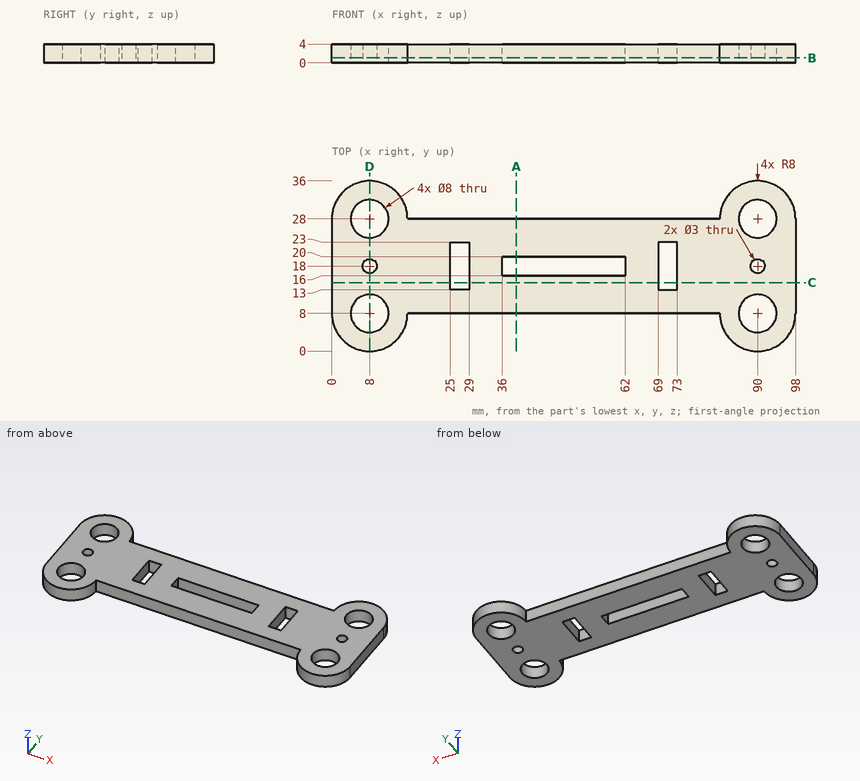
Here's the drawing with two shaded views (mm, measured from the low corner). I have some questions. Round coordinates to 2 decimals unless told otherwise and drop trailing zeros. Order: outer loops, then holes, each group sorted by start corner. A loop starts at its lowest first (then second) coordinate and runs counter-clockwise, first axis right, second up. Notation, with made-up numbers: (14, -39.5) -> (62, -39.5) arc R29 cw to (62, -5.5) -> close; hole circle Ø2 at (74.25, 51). An arc over 180 degrees is marked (long way). Return JSON: item names as keys, results as strings.
Q1. I need wall thicknesses on line 1 along X through (y, z) = (18, 2.3); line 2 along X through (y, z) = (14, 1.1); line 3 along Y through (x, z) = (8, 2.05). Which ranges of each line are inside material? Lowest first, please. Write a range as from..to.
Filled sheet:
{"line 1": "x = 0..6.5, 9.5..25, 29..36, 62..69, 73..88.5, 91.5..98", "line 2": "x = 0..25, 29..69, 73..98", "line 3": "y = 0..4, 12..16.5, 19.5..24, 32..36"}
Q2. If we section it at C-C on y = 14.5: List the corners of the cut face in (x, z) for me.
Filled sheet:
{"outline": "(0, 0) -> (25, 0) -> (25, 4) -> (0, 4) -> close; (29, 0) -> (69, 0) -> (69, 4) -> (29, 4) -> close; (73, 0) -> (98, 0) -> (98, 4) -> (73, 4) -> close"}
Q3. For pin 1 Ø1.2 at (x, z) = (26, 2.5) entering from +Y; pin 2 Ø2 at (x, z) = (71, 3) entering from -Y, each with a flat end and sliding along its axis, tell me the tip position at first contact or that it passes through.
Filled sheet:
{"pin 1": "stops at y = 28", "pin 2": "stops at y = 8"}
Q4. If we section it at D-D on x = 8: List the corners of the cut face in (y, z) for me.
Filled sheet:
{"outline": "(0, 0) -> (4, 0) -> (4, 4) -> (0, 4) -> close; (12, 0) -> (16.5, 0) -> (16.5, 4) -> (12, 4) -> close; (19.5, 0) -> (24, 0) -> (24, 4) -> (19.5, 4) -> close; (32, 0) -> (36, 0) -> (36, 4) -> (32, 4) -> close"}
Q5. If we section it at A-A on x = 39: List the corners of the cut face in (y, z) for me.
Filled sheet:
{"outline": "(8, 0) -> (16, 0) -> (16, 4) -> (8, 4) -> close; (20, 0) -> (28, 0) -> (28, 4) -> (20, 4) -> close"}
Q6. If we section it at B-B on z = 1.05: Give the number of separate pieces and of enclosed holes in the cut face, plus the area to 3 significant figures.
Filled sheet:
{"separate pieces": "1", "enclosed holes": "9", "area": "1,960 mm^2"}
